from build123d import *

# Parameters (mm, degrees)
SKETCH_1_W          = 187
SKETCH_1_H          = 2
EXTRUDE_1_DEPTH     = 4
SKETCH_2_W          = 1
SKETCH_2_H          = 4
EXTRUDE_1_2_DEPTH   = 1
FILLET_1_R          = 2
SKETCH_3_W          = 5
SKETCH_3_H          = 2
CUT_EXTRUDE_1_DEPTH = 188.053468292
FILLET_2_R          = 2


with BuildPart() as part:
    # 草图1 → Extrude 1 (new body)
    with BuildSketch(Plane.XY):
        with Locations((93.5, -1)):
            Rectangle(SKETCH_1_W, SKETCH_1_H)
    extrude(amount=EXTRUDE_1_DEPTH)

    # 草图2 → Extrude 1 2 (add)
    with BuildSketch(Plane.XZ.offset(2)):
        with Locations((0.5, 2)):
            Rectangle(SKETCH_2_W, SKETCH_2_H)
    extrude(amount=EXTRUDE_1_2_DEPTH)

    # 圆角1
    fillet_1_edges = [part.edges().sort_by_distance(p)[0] for p in [
        (0, 0, 2),
    ]]
    fillet(fillet_1_edges, radius=FILLET_1_R)

    # 草图3 → 切除-拉伸1 (cut, through all)
    with BuildSketch(Plane.XZ.offset(2)):
        with Locations((184.5, 1)):
            Rectangle(SKETCH_3_W, SKETCH_3_H)
    extrude(amount=-CUT_EXTRUDE_1_DEPTH, mode=Mode.SUBTRACT)

    # 圆角2
    fillet_2_edges = [part.edges().sort_by_distance(p)[0] for p in [
        (182, -1, 2),
    ]]
    fillet(fillet_2_edges, radius=FILLET_2_R - 0.0001)  # a hair under: the kernel refuses the full size


solid = part.part
Work out the finished part from the listing and answer in its coordinate system (mm). A direction names the side the tool comes from. Give positions to 0.01 mm unless a question says otherwise; leave off trailing zeros. Loops run counter-clockwise (first coordinate to the right, second up) from the corner with the lowest first, then second, coordinate; pieces in that order, holes last. Notation, with made-up numbers: (37.25, 73) - (43.25, 73) arc R8 cw to (43.25, 82) - close; hole circle Ø9 at (-28.5, 50.5). An arc over 180 degrees is marked (long way). Answer in a Markdown table with one row per item.
(1) Section B-B (x = 146) is taken. Give the vertices of the cut face in (y, z).
Results list:
| item | result |
|---|---|
| outline | (-2, 0) - (0, 0) - (0, 4) - (-2, 4) - close |
(2) Flat-ended cylindrical pins translate along their axes: pin 1 Ø0.5 at (y, z) = (-2.5, 1.5) entering from +X; pin 2 Ø1.2 at (x, z) = (54.5, 2.5) entering from -Y; pin 3 Ø0.6 at (x, y) = (186, -0.5) entering from -Z. Find the tip coordinate at first contact, or state that the pin passes through.
Results list:
| item | result |
|---|---|
| pin 1 | stops at x = 1 |
| pin 2 | stops at y = -2 |
| pin 3 | stops at z = 2 |
(3) A tool of negligible diameter and unlimited length cuts with its end or side. For faces 1 (the face through (93, -2, 2)), 2 (the face through (92, -1, 4)), from which of +Z, -Z, +X, -X, +Y, -Y can it reach the whole face along a straight path? Write none if from no direction.
Results list:
| item | result |
|---|---|
| face 1 | +Z, -Z, +X, -Y |
| face 2 | +Z, +X, -X, +Y, -Y |
(4) Section A-A (z = 3.25) is taken. Give the vertices of the cut face in (x, y), and give its area (3 significant figures).
Results list:
| item | result |
|---|---|
| outline | (0, -3) - (1, -3) - (1, -2) - (187, -2) - (187, 0) - (2, 0) arc R2 ccw to (0, -2) - close |
| area | 374 mm² |
(5) Consider L1, parallel to Y at x = 117, z = 1.45; L2, parallel to X at y = -2.4, z = 2; L3, parallel to X at y = -1.8, z = 2.45. Determine where each line is inside the solid, lowest interval first. Write a range as [from, to].
Results list:
| item | result |
|---|---|
| L1 | y = [-2, 0] |
| L2 | x = [0, 1] |
| L3 | x = [0.01, 187] |
